Work out the finished part from the listing and answer in its coordinate system (mm). Coordinates: 2 decimals unless noted, no trailing zeros. Order: outer loops, then holes, each group sorted by start corner. A loop starts at its lowest first (then second) coordinate and runs counter-clockwise, first axis right, second up. Notation, with made-up numbers: (1, 45.5) - (33, 45.5) arc R16 ccw to (33, 69.5) - close; hole circle Ø6 at (-15.75, 87.5). An arc over 180 degrees is marked (long way). Use CSV: the item, a comma, the result in double quotes. Start each with the question number.
from build123d import *

# Parameters (mm, degrees)
F0_R     = 4
F1_DEPTH = 2.5


with BuildPart() as f1:
    # F0 (on Front) → F1 (new body)
    with BuildSketch(Plane.XZ):
        with BuildLine():
            ThreePointArc((0, 10), (2.928932, 2.928932), (10, 0))
            Line((10, 0), (540, 0))
            ThreePointArc((540, 0), (547.071068, 2.928932), (550, 10))
            Line((550, 10), (550, 210))
            ThreePointArc((550, 210), (547.071068, 217.071068), (540, 220))
            Line((540, 220), (10, 220))
            ThreePointArc((10, 220), (2.928932, 217.071068), (0, 210))
            Line((0, 210), (0, 10))
        make_face()
        with Locations((14, 14)):
            Circle(F0_R, mode=Mode.SUBTRACT)
        with BuildLine():
            Line((220.000318, 40.079729), (220.000318, 179.920271))
            ThreePointArc((220.000318, 179.920271), (229.960135, 189.999921), (240, 180))
            Line((240, 180), (240, 40))
            ThreePointArc((240, 40), (230.039865, 30.000079), (220.000318, 39.920271))
            ThreePointArc((220.000318, 39.920271), (220, 40), (220.000318, 40.079729))
        make_face(mode=Mode.SUBTRACT)
        with Locations((275, 14)):
            Circle(F0_R, mode=Mode.SUBTRACT)
        with Locations((536, 14)):
            Circle(F0_R, mode=Mode.SUBTRACT)
        with BuildLine():
            Line((265.000318, 40.079729), (265.000318, 179.920271))
            ThreePointArc((265.000318, 179.920271), (274.960135, 189.999921), (285, 180))
            Line((285, 180), (285, 40))
            ThreePointArc((285, 40), (275.039865, 30.000079), (265.000318, 39.920271))
            ThreePointArc((265.000318, 39.920271), (265, 40), (265.000318, 40.079729))
        make_face(mode=Mode.SUBTRACT)
        with BuildLine():
            ThreePointArc((40.000318, 179.920271), (49.960135, 189.999921), (60, 180))
            Line((60, 180), (60, 40))
            ThreePointArc((60, 40), (50.039865, 30.000079), (40.000318, 39.920271))
            ThreePointArc((40.000318, 39.920271), (40, 40), (40.000318, 40.079729))
            Line((40.000318, 40.079729), (40.000318, 179.920271))
        make_face(mode=Mode.SUBTRACT)
        with BuildLine():
            Line((85.000318, 40.079729), (85.000318, 179.920271))
            ThreePointArc((85.000318, 179.920271), (94.960135, 189.999921), (105, 180))
            Line((105, 180), (105, 40))
            ThreePointArc((105, 40), (95.039865, 30.000079), (85.000318, 39.920271))
            ThreePointArc((85.000318, 39.920271), (85, 40), (85.000318, 40.079729))
        make_face(mode=Mode.SUBTRACT)
        with BuildLine():
            Line((130.000318, 40.079729), (130.000318, 179.920271))
            ThreePointArc((130.000318, 179.920271), (139.960135, 189.999921), (150, 180))
            Line((150, 180), (150, 40))
            ThreePointArc((150, 40), (140.039865, 30.000079), (130.000318, 39.920271))
            ThreePointArc((130.000318, 39.920271), (130, 40), (130.000318, 40.079729))
        make_face(mode=Mode.SUBTRACT)
        with BuildLine():
            Line((175.000318, 40.079729), (175.000318, 179.920271))
            ThreePointArc((175.000318, 179.920271), (184.960135, 189.999921), (195, 180))
            Line((195, 180), (195, 40))
            ThreePointArc((195, 40), (185.039865, 30.000079), (175.000318, 39.920271))
            ThreePointArc((175.000318, 39.920271), (175, 40), (175.000318, 40.079729))
        make_face(mode=Mode.SUBTRACT)
        with Locations((14, 206)):
            Circle(F0_R, mode=Mode.SUBTRACT)
        with BuildLine():
            Line((310.000318, 40.079729), (310.000318, 179.920271))
            ThreePointArc((310.000318, 179.920271), (319.960135, 189.999921), (330, 180))
            Line((330, 180), (330, 40))
            ThreePointArc((330, 40), (320.039865, 30.000079), (310.000318, 39.920271))
            ThreePointArc((310.000318, 39.920271), (310, 40), (310.000318, 40.079729))
        make_face(mode=Mode.SUBTRACT)
        with BuildLine():
            Line((355.000318, 40.079729), (355.000318, 179.920271))
            ThreePointArc((355.000318, 179.920271), (364.960135, 189.999921), (375, 180))
            Line((375, 180), (375, 40))
            ThreePointArc((375, 40), (365.039865, 30.000079), (355.000318, 39.920271))
            ThreePointArc((355.000318, 39.920271), (355, 40), (355.000318, 40.079729))
        make_face(mode=Mode.SUBTRACT)
        with BuildLine():
            Line((400.000318, 40.079729), (400.000318, 179.920271))
            ThreePointArc((400.000318, 179.920271), (409.960135, 189.999921), (420, 180))
            Line((420, 180), (420, 40))
            ThreePointArc((420, 40), (410.039865, 30.000079), (400.000318, 39.920271))
            ThreePointArc((400.000318, 39.920271), (400, 40), (400.000318, 40.079729))
        make_face(mode=Mode.SUBTRACT)
        with BuildLine():
            Line((445.000318, 40.079729), (445.000318, 179.920271))
            ThreePointArc((445.000318, 179.920271), (454.960135, 189.999921), (465, 180))
            Line((465, 180), (465, 40))
            ThreePointArc((465, 40), (455.039865, 30.000079), (445.000318, 39.920271))
            ThreePointArc((445.000318, 39.920271), (445, 40), (445.000318, 40.079729))
        make_face(mode=Mode.SUBTRACT)
        with BuildLine():
            Line((490.000318, 40.079729), (490.000318, 179.920271))
            ThreePointArc((490.000318, 179.920271), (499.960135, 189.999921), (510, 180))
            Line((510, 180), (510, 40))
            ThreePointArc((510, 40), (500.039865, 30.000079), (490.000318, 39.920271))
            ThreePointArc((490.000318, 39.920271), (490, 40), (490.000318, 40.079729))
        make_face(mode=Mode.SUBTRACT)
        with Locations((275, 206)):
            Circle(F0_R, mode=Mode.SUBTRACT)
        with Locations((536, 206)):
            Circle(F0_R, mode=Mode.SUBTRACT)
    extrude(amount=F1_DEPTH)


solid = f1.part
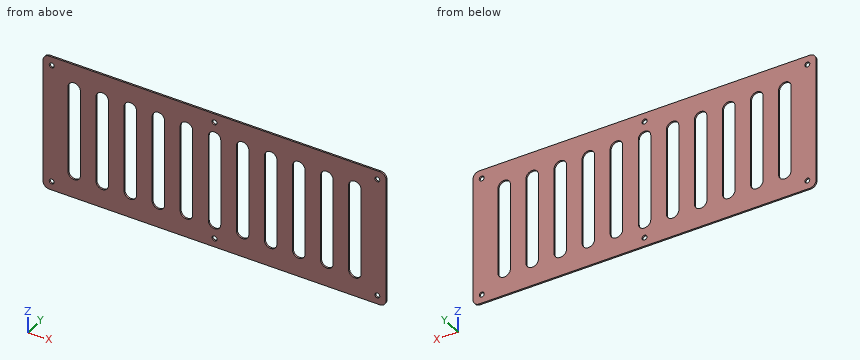
1) Straight lines are drawn through the part: line 1 (Z direction, x = 275, y = -0.55); line 2 (Z direction, x = 14, y = -1.5); line 3 (Z direction, x = 499, y = -1.9). For each, find the intervals that lie inside material, in ascending order. Write a range as [from, to].
2) The part is cut by section B-B on z = 121.5. State how many separate pieces and enclosed holes the cut face has, plus the area to 3 significant figures.
3) The part is cut by section A-A on x = 95. Determine the outline of the cut face in (y, z).
Answer key:
1,line 1,"[0, 10], [18, 30], [190, 202], [210, 220]"
1,line 2,"[0, 10], [18, 202], [210, 220]"
1,line 3,"[0, 30.05], [189.95, 220]"
2,separate pieces,"12"
2,enclosed holes,"0"
2,area,"825 mm^2"
3,outline,"(-2.5, 0) - (0, 0) - (0, 30) - (-2.5, 30) - close; (-2.5, 190) - (0, 190) - (0, 220) - (-2.5, 220) - close"
